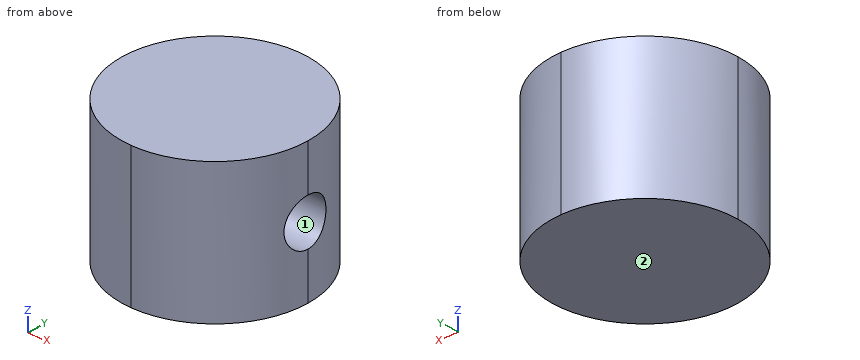
```python
from build123d import *

# Parameters (mm, degrees)
SKETCH1_W           = 16
SKETCH1_H           = 16
BOSS_EXTRUDE1_DEPTH = 12
CUT_EXTRUDE1_DEPTH  = 13
SKETCH2_R           = 2
CUT_EXTRUDE2_DEPTH  = 10


with BuildPart() as part:
    # Sketch1 → Boss-Extrude1 (new body)
    with BuildSketch(Plane.XY):
        with Locations((-14.67401686, 4.154520967)):
            Rectangle(SKETCH1_W, SKETCH1_H)
    extrude(amount=BOSS_EXTRUDE1_DEPTH)

    # Sketch3 → Cut-Extrude1 (cut)
    with BuildSketch(Plane.XY.offset(12)):
        with BuildLine():
            Line((-6.67401686, 12.154520967), (-14.67401686, 12.154520967))
            ThreePointArc((-14.67401686, 12.154520967), (-9.017162611, 9.811375216), (-6.67401686, 4.154520967))
            Line((-6.67401686, 4.154520967), (-6.67401686, 12.154520967))
        make_face()
        with BuildLine():
            Line((-6.67401686, -3.845479033), (-6.67401686, 4.154520967))
            ThreePointArc((-6.67401686, 4.154520967), (-9.017162611, -1.502333283), (-14.67401686, -3.845479033))
            Line((-14.67401686, -3.845479033), (-6.67401686, -3.845479033))
        make_face()
        with BuildLine():
            Line((-14.67401686, 12.154520967), (-22.67401686, 12.154520967))
            Line((-22.67401686, 12.154520967), (-22.67401686, 4.154520967))
            ThreePointArc((-22.67401686, 4.154520967), (-20.33087111, 9.811375216), (-14.67401686, 12.154520967))
        make_face()
        with BuildLine():
            ThreePointArc((-14.67401686, -3.845479033), (-20.33087111, -1.502333283), (-22.67401686, 4.154520967))
            Line((-22.67401686, 4.154520967), (-22.67401686, -3.845479033))
            Line((-22.67401686, -3.845479033), (-14.67401686, -3.845479033))
        make_face()
    extrude(amount=-CUT_EXTRUDE1_DEPTH, mode=Mode.SUBTRACT)

    # Sketch2 → Cut-Extrude2 (cut)
    with BuildSketch(Plane(origin=(-6.67401686, 0, 0), x_dir=(0, 0, -1), z_dir=(1, 0, 0))):
        with Locations(Location((-6, 4.154520967, 0), (0, 0, 90))):
            Circle(SKETCH2_R)
    extrude(amount=-CUT_EXTRUDE2_DEPTH, mode=Mode.SUBTRACT)


solid = part.part
```
Geometry: final body of the model. Coordinates: model frame, mm. Face numbers are marked on the shaded views. Round coordinates to 2 decimals unless told otherwise and drop trailing zeros. Order: outer loops, then holes, each group sorted by start corner. A loop starts at its lowest first (then second) coordinate and runs counter-clockwise, first axis right, second up. Notation, with made-up numbers: (-19.5, -30) -> (39.5, -30) arc R9 cw to (39.5, -13) -> close; hole circle Ø3 at (-13, 72). An arc over 180 degrees is marked (long way). Use CSV: the item, a comma, the result in double quotes. Start each with the question number.
1) Section D-D (z = 10.25). Return the cut outline in (x, y).
2) Section C-C (x = -13.5). Return the cut outline in (y, z).
3) Section A-A (z = 4.75). Return the cut outline in (x, y), and give its area (3 significant figures).
4) First-contact query: pin 1 Ø5 at (x, z) = (-17, 4) entering from +Y; pin 2 Ø5 at (y, z) = (-1.5, 4.5) entering from -X. Flat tips, straight axial feed; report the tip coordinate or a pass-through.
5) Draft query along Y for the marked faces 1 and 2. Return one class per face: +Y half, -Y half, draft (parallel to the pull), parting line (faces both ways), or undercut.
6) Section B-B (y = 5.75). Return the cut outline in (x, z), and give its area (3 significant figures).
7) Material intervals for line 1 along Y through (x, z) = (-14.75, 3.25); line 2 along Y through (x, z) = (-8.5, 5); line 3 along Y through (x, z) = (-10.5, 6), sorted ascending. Write a range as from..to.
Returned:
1,outline,"circle Ø16 at (-14.67, 4.15)"
2,outline,"(-3.76, 0) -> (12.07, 0) -> (12.07, 12) -> (-3.76, 12) -> close; hole circle Ø4 at (4.15, 6)"
3,outline,"(-16.67, 2.59) -> (-16.67, 5.72) -> (-6.83, 5.72) arc R8 ccw (long way) to (-6.83, 2.59) -> close"
3,area,"170 mm²"
4,pin 1,"stops at y = 12.15"
4,pin 2,"stops at x = -22.03"
5,face 1,"undercut"
5,face 2,"draft"
6,outline,"(-22.51, 0) -> (-6.83, 0) -> (-6.83, 4.79) -> (-16.67, 4.79) -> (-16.67, 7.21) -> (-6.83, 7.21) -> (-6.83, 12) -> (-22.51, 12) -> close"
6,area,"164 mm²"
7,line 1,"y = -3.85..12.15"
7,line 2,"y = -0.93..2.42, 5.89..9.24"
7,line 3,"y = -2.67..2.15, 6.15..10.98"
